Autodesk Inventor part; units mm, degrees
ref_plane "YZ Plane" through (0, 0, 0) normal (1, 0, 0) x (0, 1, 0)
ref_plane "XZ Plane" through (0, 0, 0) normal (0, 1, 0) x (-1, 0, 0)
ref_plane "XY Plane" through (0, 0, 0) normal (0, 0, 1) x (1, 0, 0)
sketch "Sketch1" plane through (0, 0, 0) normal (0, 1, 0) x (-1, 0, 0)
  line L0 (0, 0) -> (96.52, 0)
  line L1 (96.52, 0) -> (96.52, -112.7)
  line L2 (96.52, -112.7) -> (0, -112.7)
  line L3 (0, -112.7) -> (0, 0)
  dimension "d0" = 96.52
  dimension "d1" = 112.7
extrude "Extrusion1" add sketch "Sketch1" along normal blind 10.16
sketch "Sketch2" plane through (0, 10.16, 0) normal (0, 1, 0) x (1, 0, 0)
  line L0 (-96.52, 112.7) -> (-96.52, 0) construction
  line L1 (0, 0) -> (0, 112.7) construction
  line L2 (-96.52, 0) -> (0, 112.7) construction
  line L3 (0, 112.7) -> (-96.52, 112.7) construction
  line L4 (-96.52, 112.7) -> (0, 0) construction
  line L5 (-93.98, 4.28) -> (-2.54, 4.28)
  line L6 (-2.54, 4.28) -> (-2.54, 108.42)
  line L7 (-2.54, 108.42) -> (-93.98, 108.42)
  line L8 (-93.98, 108.42) -> (-93.98, 4.28)
  line L9 (-93.98, 4.28) -> (-2.54, 108.42) construction
  line L10 (-2.54, 4.28) -> (-93.98, 108.42) construction
  point P0 (-48.26, 56.35)
  dimension "d4" = 91.44
  dimension "d5" = 104.14
extrude "Jetson Cavity" cut sketch "Sketch2" against normal blind 3.81
sketch "Sketch3" plane through (0, 0, 0) normal (0, -1, 0) x (1, 0, 0)
  line L0 (0, -19.05) -> (6.35, -19.05)
  line L1 (6.35, -19.05) -> (6.35, -25.4)
  line L2 (6.35, -25.4) -> (0, -25.4)
  circle A0 centre (3.175, -22.225) radius 1.7
  line L3 (6.35, -25.4) -> (0, -19.05) construction
  line L4 (6.35, -19.05) -> (0, -25.4) construction
  line L5 (0, 0) -> (0, -112.7) construction
  line L6 (0, -56.35) -> (-96.52, -56.35) construction
  line L7 (-96.52, -112.7) -> (-96.52, 0) construction
  line L8 (0, -112.7) -> (-96.52, -112.7) construction
  line L9 (-48.26, -112.7) -> (-48.26, 0) construction
  line L10 (-96.52, 0) -> (0, 0) construction
  line L11 (-96.52, 0) -> (-96.52, -112.7) construction
  line L12 (0, 0) -> (27.0549, 0) construction
  line L13 (0, -19.05) -> (0, -25.4)
  line L14 (-96.52, -19.05) -> (-102.87, -19.05)
  line L15 (-102.87, -19.05) -> (-102.87, -25.4)
  line L16 (-102.87, -25.4) -> (-96.52, -25.4)
  circle A1 centre (-99.695, -22.225) radius 1.7
  line L17 (-102.87, -25.4) -> (-96.52, -19.05) construction
  line L18 (-102.87, -19.05) -> (-96.52, -25.4) construction
  line L19 (-96.52, 0) -> (-96.52, -112.7) construction
  line L20 (-96.52, -19.05) -> (-96.52, -25.4)
  line L21 (0, -93.65) -> (6.35, -93.65)
  line L22 (6.35, -93.65) -> (6.35, -87.3)
  line L23 (6.35, -87.3) -> (0, -87.3)
  circle A2 centre (3.175, -90.475) radius 1.7
  line L24 (6.35, -87.3) -> (0, -93.65) construction
  line L25 (6.35, -93.65) -> (0, -87.3) construction
  line L26 (0, -112.7) -> (0, 0) construction
  line L27 (0, -93.65) -> (0, -87.3)
  line L28 (-96.52, -93.65) -> (-96.52, -87.3)
  circle A3 centre (-99.695, -90.475) radius 1.7
  line L29 (-102.87, -87.3) -> (-96.52, -93.65) construction
  line L30 (-102.87, -93.65) -> (-102.87, -87.3)
  line L31 (-102.87, -87.3) -> (-96.52, -87.3)
  line L32 (-102.87, -93.65) -> (-96.52, -87.3) construction
  line L33 (-96.52, -93.65) -> (-102.87, -93.65)
  line L34 (-77.47, 6.35) -> (-71.12, 6.35)
  line L35 (-71.12, 6.35) -> (-71.12, 0)
  line L36 (-71.12, 0) -> (-77.47, 0)
  line L37 (-77.47, 0) -> (-77.47, 6.35)
  line L38 (-77.47, 6.35) -> (-71.12, 0) construction
  line L39 (-71.12, 6.35) -> (-77.47, 0) construction
  circle A4 centre (-74.295, 3.175) radius 1.7
  line L40 (-96.52, 0) -> (-96.52, 26.4088) construction
  line L41 (-19.05, 6.35) -> (-25.4, 6.35)
  line L42 (-25.4, 6.35) -> (-25.4, 0)
  line L43 (-25.4, 0) -> (-19.05, 0)
  line L44 (-19.05, 0) -> (-19.05, 6.35)
  line L45 (-19.05, 6.35) -> (-25.4, 0) construction
  line L46 (-25.4, 6.35) -> (-19.05, 0) construction
  circle A5 centre (-22.225, 3.175) radius 1.7
  line L47 (-77.47, -119.05) -> (-71.12, -119.05)
  line L48 (-71.12, -119.05) -> (-71.12, -112.7)
  line L49 (-71.12, -112.7) -> (-77.47, -112.7)
  line L50 (-77.47, -112.7) -> (-77.47, -119.05)
  line L51 (-77.47, -119.05) -> (-71.12, -112.7) construction
  line L52 (-71.12, -119.05) -> (-77.47, -112.7) construction
  circle A6 centre (-74.295, -115.875) radius 1.7
  line L53 (-25.4, -112.7) -> (-19.05, -112.7)
  line L54 (-25.4, -119.05) -> (-25.4, -112.7)
  circle A7 centre (-22.225, -115.875) radius 1.7
  line L55 (-19.05, -112.7) -> (-19.05, -119.05)
  line L56 (-19.05, -119.05) -> (-25.4, -112.7) construction
  line L57 (-25.4, -119.05) -> (-19.05, -112.7) construction
  line L58 (-19.05, -119.05) -> (-25.4, -119.05)
  point P0 (-77.47, 3.175)
  point P1 (-19.05, 3.175)
  point P2 (-77.47, -115.875)
  point P3 (-19.05, -115.875)
  dimension "d10" = 3.4
  dimension "d28" = 6.35
  dimension "d29" = 6.35
  dimension "d30" = 19.05
  dimension "d31" = 6.35
  dimension "d32" = 6.35
  dimension "d33" = 3.4
  dimension "d34" = 19.05
extrude "Screws" add sketch "Sketch3" against normal blind 3.175
sketch "Sketch5" plane through (0, 0, 0) normal (0, -1, 0) x (1, 0, 0)
  line L0 (-102.87, 6.35) -> (-71.12, 6.35)
  line L1 (-71.12, 6.35) -> (-71.12, -25.4)
  line L2 (-71.12, -25.4) -> (-102.87, -25.4)
  line L3 (-102.87, -25.4) -> (-102.87, 6.35)
  line L4 (-71.12, 6.35) -> (-77.47, 6.35)
  line L5 (-102.87, -19.05) -> (-102.87, -25.4)
  line L6 (-96.52, -19.05) -> (-96.52, 0)
  line L7 (-96.52, 0) -> (-77.47, 0)
  line L8 (-102.87, 6.35) -> (6.35, 6.35)
  line L9 (6.35, 6.35) -> (6.35, -119.05)
  line L10 (6.35, -119.05) -> (-102.87, -119.05)
  line L11 (-102.87, -119.05) -> (-102.87, 6.35)
  line L12 (6.35, -93.65) -> (6.35, -87.3)
  line L13 (-25.4, -119.05) -> (-19.05, -119.05)
  dimension "d35" = 25.4
  dimension "d36" = 25.4
extrude "Extrusion5" cut sketch "Sketch5" against normal through all contours L8 L9 L10 L11 L2 L1
equation "\"d10\" = m3_clearance"
equation "\"d33\" = m3_clearance"
equation "\"m3_heat_set_insert\" = 4"
equation "\"m3_clearance\" = 3.4"
equation "\"m3_heat_set_depth\" = 7"
equation "\"robot_diameter\" = 354"
equation "\"hardboard_thickness\" = 5"
properties part number "jetson_orin_nano_holder_corner_2"
The listing builds one solid part. Answer for the finished solid, in the listing's coordinates (mm). A direction names the side the tool comes from. Give positions to 0.01 mm unless a question says otherwise; leave off trailing zeros. Write each loop counter-clockwise with the first axis right and the second up, starting at its lowest first coordinate (ties: lowest second). Pieces come first, ordered by that corner, then holes. Notation, with made-up numbers: (55.5, -30.5) - (82.5, -30.5) arc R17 ccw to (82.5, -12.5) - close; hole circle Ø3 at (-40, -6). An arc over 180 degrees is marked (long way). One line per question, with ' | ' between items. Start each with the question number.
1. Given P1, Ø5.5, axis at x = -74.295, z = 3.175, coming from the -Y side; P2, Ø10.5, axis at x = -82.5, z = -19.5, coming from the +Y side; P3, Ø1, axis at y = 2, z = 3, coming from the -X side; P4, Ø1, axis at x = -99, y = 1, coming from the +Z side, each flat-ended and moving along its own axis, determine where each tip first touches the part or whether it passes through.
2. Section C-C, the plane z = -10 is taken. Determine the outline of the cut face in (x, y).
3. Straight lines are drawn through the part: line 1 (Z direction, x = -77.5, y = 3.5); line 2 (X direction, y = 7.75, z = -17.5); line 3 (X direction, y = 2.5, z = -5). For each, find the intervals that lie inside material, in ascending order.
4. Section A-A, the plane x = -77 is taken. Determine the outline of the cut face in (y, z) (3 decimals), then the cut area to 3 significant figures.
5. For faces 5 (the face through (-72.9, 3.175, 1.8)), 6 (the face through (-98, 3.175, -21)), 7 (the face through (-83, 8, -4.28)), 8 (the face through (-77.47, 2, 3)), determine the directions among +Z, -Z, +X, -X, +Y, -Y from which every point of the face is accessible in a straight line to the end or side of a thin tool.
6. Section D-D, the plane x = -90 is taken. Determine the outline of the cut face in (y, z).
7. Determine the mould class of faces 1 (the face through (-101.044, 1.565, -23.259)), 2 (the face through (-100, 2, -19.05)), 3 (the face through (-87, 3, -25.4)), 4 (the face through (-71.12, 4, -9)) for opening direction Z: +Z half, -Z half, draft (parallel to the pull), parting line (faces both ways), or undercut.
8. Section B-B, the plane y = 2.75 is taken. Determine the outline of the cut face in (x, z) (3 decimals).
Result:
1) P1: stops at y = 0 | P2: stops at y = 6.35 | P3: stops at x = -77.47 | P4: stops at z = -19.05
2) outline: (-96.52, 0) - (-71.12, 0) - (-71.12, 6.35) - (-93.98, 6.35) - (-93.98, 10.16) - (-96.52, 10.16) - close
3) line 1: z = -25.4 to 0 | line 2: x = -96.52 to -93.98 | line 3: x = -96.52 to -71.12
4) outline: (0, -25.4) - (6.35, -25.4) - (6.35, -4.28) - (10.16, -4.28) - (10.16, 0) - (3.175, 0) - (3.175, 6.35) - (0, 6.35) - close | area: 198 mm2
5) face 5: +Z, +X, -X, +Y | face 6: +Z, -Z, -X, +Y | face 7: -Z, +X, +Y | face 8: +Z, -X, +Y, -Y
6) outline: (0, -25.4) - (6.35, -25.4) - (6.35, -4.28) - (10.16, -4.28) - (10.16, 0) - (0, 0) - close
7) face 1: undercut | face 2: +Z half | face 3: -Z half | face 4: draft
8) outline: (-102.87, -25.4) - (-71.12, -25.4) - (-71.12, 6.35) - (-77.47, 6.35) - (-77.47, 0) - (-96.52, 0) - (-96.52, -19.05) - (-102.87, -19.05) - close; hole circle Ø3.4 at (-99.695, -22.225); hole circle Ø3.4 at (-74.295, 3.175)
